Autodesk Fusion 360 part; units mm, degrees
sketch "Top" plane through (0, 0, 0) normal (0, 0, 1) x (1, 0, 0)
  line L0 (0, 0) -> (40, 0)
  line L1 (40, 0) -> (40, 50)
  line L2 (40, 50) -> (0, 50)
  line L3 (0, 50) -> (0, 0)
  circle A0 centre (20, 25) radius 8.1
  dimension "d6" = 40
  dimension "d7" = 50
  dimension "d11" = 16.2
  dimension "d12" = 25
  dimension "d13" = 20
extrude "Extrude1" add sketch "Top" along normal blind 10 contours L0 L1 L2 L3 | A0
extrude "Extrude2" cut sketch "Top" along normal blind 20 contours A0
sketch "Sketch2" plane through (40, 0, 0) normal (1, 0, 0) x (0, 1, 0)
  line L0 (0, 0) -> (50, 0)
  line L1 (50, 0) -> (50, 10)
  line L2 (50, 10) -> (0, 10)
  line L3 (0, 10) -> (0, 0)
  circle A0 centre (5, 5) radius 3.75
  circle A1 centre (45, 5) radius 3.75
  dimension "d16" = 7.5
  dimension "d17" = 7.5
  dimension "d18" = 5
  dimension "d19" = 5
  dimension "d20" = 5
  dimension "d21" = 5
extrude "Extrude3" cut sketch "Sketch2" against normal blind 50 contours A0
extrude "Extrude4" cut sketch "Sketch2" against normal blind 50 contours A1
equation "length = 50 mm"
equation "width = 40 mm"
equation "thickness = 10 mm"
equation "extra = 10 mm"
equation "fit_gap = 0.2 mm"
equation "d6 = width"
equation "d7 = length"
equation "d8 = thickness"
equation "bearing_8155_outer_radius = 8 mm"
equation "d11 = ( bearing_8155_outer_radius * 2 ) + fit_gap"
equation "d12 = length / 2"
equation "d13 = width / 2"
equation "d14 = thickness + extra"
equation "d16 = 3 * thickness / 4"
equation "d17 = 3 * thickness / 4"
equation "d18 = thickness / 2"
equation "d19 = thickness / 2"
equation "d20 = thickness / 2"
equation "d21 = thickness / 2"
For this review, take the finished solid that the model builds, in its own axes (mm). Give positions to 0.01 mm unless a question says otherwise; leave off trailing zeros. Order: outer loops, then holes, each group sorted by start corner. A loop starts at its lowest first (then second) coordinate and runs counter-clockwise, first axis right, second up. Notation, with made-up numbers: M 39,38.5 L 67,38.5 A28 ccw 67,70.5 Z; hole C -21.5,-18.5 d11. An arc over 180 degrees is marked long. Answer in a Markdown table with one row per item. Add a question column.
(1) Wall thickness on probe 1 along Z at (x, y) = (13.5, 5); probe 2 along X at (y, z) = (25, 7.5); probe 3 along Y at (x, z) = (20, 2.75): over which ranges is each line inside the solid? List them lowest first. Write a range as [from, to].
(2) Consider section A-A on x = 20. State the section outline as (y, z) points.
(3) Consider section D-D on x = 6. State the section outline as (y, z) points.
(4) For pin 1 (13 mm diameter, centred on x = 20, y = 25, fed in from +Z); pin 2 (4 mm diameter, centred on x = 13.5, z = 3, fed in from -Y), all flat-tipped, find the tip position at first contact; note any pin that passes through.
(5) Mouldability with a two-part tool opening along X and no side actions: class faces 1 (the face through (14.03, 19.526, 4.93)), 2 (the face through (0, 25, 5)), 3 (the face through (29, 25, 10)) as +X half, -X half, draft (parallel to the pull), parting line (faces both ways), or undercut.
(6) Consider section B-B on y = 25. State the section outline as (x, z) points, and give its area (3 significant figures).
(7) Consider section C-C on z = 6.5. State the section outline as (x, y) points, and give its area (3 significant figures).
Evaluation:
| question | item | result |
|---|---|---|
| 1 | probe 1 | z = [0, 1.25], [8.75, 10] |
| 1 | probe 2 | x = [0, 11.9], [28.1, 40] |
| 1 | probe 3 | y = [0, 2], [8, 16.9], [33.1, 42], [48, 50] |
| 2 | outline | M 0,0 L 16.9,0 L 16.9,10 L 0,10 Z; M 33.1,0 L 50,0 L 50,10 L 33.1,10 Z; hole C 5,5 d7.5; hole C 45,5 d7.5 |
| 3 | outline | M 0,0 L 50,0 L 50,10 L 0,10 Z; hole C 5,5 d7.5; hole C 45,5 d7.5 |
| 4 | pin 1 | passes through |
| 4 | pin 2 | stops at y = 0 |
| 5 | face 1 | undercut |
| 5 | face 2 | -X half |
| 5 | face 3 | draft |
| 6 | outline | M 0,0 L 11.9,0 L 11.9,10 L 0,10 Z; M 28.1,0 L 40,0 L 40,10 L 28.1,10 Z |
| 6 | area | 238 mm^2 |
| 7 | outline | M 0,0 L 40,0 L 40,1.56 L 0,1.56 Z; M 0,8.44 L 40,8.44 L 40,41.56 L 0,41.56 Z; M 0,48.44 L 40,48.44 L 40,50 L 0,50 Z; hole C 20,25 d16.2 |
| 7 | area | 1,240 mm^2 |
